Work out the finished part from the listing and answer in its coordinate system (mm). Round coordinates to 2 decimals unless told otherwise and drop trailing zeros. Order: outer loops, then holes, each group sorted by start corner. A loop starts at its lowest first (then second) coordinate and runs counter-clockwise, first axis right, second up. Notation, with made-up numbers: M 41.25,58 L 45.25,58 A17 cw 45.25,89 Z; hole C 65,18 d3. An arc over 180 degrees is marked long. Return JSON: item names as keys, results as strings.
from build123d import *

# Parameters (mm, degrees)
F0_W           = 144.8953971267
F0_H           = 132.3546804488
F1_DEPTH       = 25
F3_W           = 52.6192765683
F3_H           = 54.747434333
F4_DEPTH       = 25
F6_D           = 10
F6_DEPTH       = 50
F6_CBORE_D     = 10
F6_CBORE_DEPTH = 5
F6_TIP         = 3.0043030951


with BuildPart() as f1:
    # F0 (on Front) → F1 (new body)
    with BuildSketch(Plane.XZ):
        with Locations((-90.7013751566, -26.4289211482)):
            Rectangle(F0_W, F0_H)
    extrude(amount=F1_DEPTH)


with BuildPart() as f4:
    # F3 (on Front) → F4 (new body)
    with BuildSketch(Plane.XZ):
        with Locations((-49.9591687694, 10.3274388239)):
            Rectangle(F3_W, F3_H)
    extrude(amount=F4_DEPTH)

    # F6
    with Locations(Plane.XZ.offset(25)):
        with Locations((-49.1547472775, 10.3621119633)):
            CounterBoreHole(F6_D / 2, F6_CBORE_D / 2, F6_CBORE_DEPTH, depth=F6_DEPTH)
            with Locations((0, 0, -(F6_DEPTH + F6_TIP / 2))):  # 118° drill point
                Cone(0, F6_D / 2, F6_TIP, mode=Mode.SUBTRACT)


solid = f4.part
Item 1: The mould has two halves that part along X. Classify faces 1 (the flat face through (-23.65, -12, 10)), 2 (the flat face through (-56, 0, 11)), 3 (the cylindrical face through (-48.07, -12.32, 5.48)): pulls with the +X half, pulls with the -X half, needs draft (parallel to the pull), parting line crosses it, or undercut.
Output:
{"face 1": "pulls with the +X half", "face 2": "needs draft", "face 3": "undercut"}
Item 2: Find section C-C (y = -10). Determine the outline of the cut face in (x, z).
Output:
{"outline": "M -76.27,-17.05 L -23.65,-17.05 L -23.65,37.7 L -76.27,37.7 Z; hole C -49.15,10.36 d10"}
Item 3: Find section A-A (z = 12). Determine the outline of the cut face in (x, y), plus the area to 3 significant figures.
Output:
{"outline": "M -76.27,-25 L -53.88,-25 L -53.88,0 L -76.27,0 Z; M -44.43,-25 L -23.65,-25 L -23.65,0 L -44.43,0 Z", "area": "1,080 mm^2"}
Item 4: Consider line 1 along Z through (x, y) = (-45.5, -17.25); line 2 along Z through (x, y) = (-50.5, -16.5); line 3 along X through (y, z) = (-3, 9.5). Determine where each line is inside the solid, lowest interval first. Write a range as [from, to].
Output:
{"line 1": "z = [-17.05, 6.95], [13.77, 37.7]", "line 2": "z = [-17.05, 5.55], [15.18, 37.7]", "line 3": "x = [-76.27, -54.08], [-44.23, -23.65]"}
Item 5: Find section B-B (x = -52.5). Determine the outline of the cut face in (y, z).
Output:
{"outline": "M -25,-17.05 L 0,-17.05 L 0,6.65 L -25,6.65 Z; M -25,14.08 L 0,14.08 L 0,37.7 L -25,37.7 Z"}
